from build123d import *

# Parameters (mm, degrees)
F0_W          = 203.2
F0_H          = 2032
F0_W_2        = 171.45
F0_H_2        = 320.1458333333
F1_DEPTH      = 22.225
F1_DEPTH_BACK = 22.225
F2_W          = 171.45
F2_H          = 320.1458333333
F3_DEPTH      = 21.59
F3_DEPTH_BACK = 21.59


with BuildPart() as f1:
    # F0 (on Front) → F1 (new body, two sides)
    with BuildSketch(Plane.XZ) as f1_sk:
        with Locations((101.6, 1016)):
            Rectangle(F0_W, F0_H)
        with Locations((101.6, 175.9479166667)):
            Rectangle(F0_W_2, F0_H_2, mode=Mode.SUBTRACT)
        with Locations((101.6, 511.96875)):
            Rectangle(F0_W_2, F0_H_2, mode=Mode.SUBTRACT)
        with Locations((101.6, 847.9895833333)):
            Rectangle(F0_W_2, F0_H_2, mode=Mode.SUBTRACT)
        with Locations((101.6, 1184.0104166667)):
            Rectangle(F0_W_2, F0_H_2, mode=Mode.SUBTRACT)
        with Locations((101.6, 1520.03125)):
            Rectangle(F0_W_2, F0_H_2, mode=Mode.SUBTRACT)
        with Locations((101.6, 1856.0520833333)):
            Rectangle(F0_W_2, F0_H_2, mode=Mode.SUBTRACT)
    extrude(amount=F1_DEPTH)
    extrude(f1_sk.sketch, amount=-F1_DEPTH_BACK)

    # F2 (on Front) → F3 (join, two sides)
    with BuildSketch(Plane.XZ) as f3_sk:
        with Locations((101.6, 1520.03125)):
            Rectangle(F2_W, F2_H)
        with BuildLine():
            Line((40.0148101771, 1504.2365351889), (122.7722068767, 1592.3491351889))
            ThreePointArc((122.7722068767, 1592.3491351889), (127.2601313551, 1592.4897903562), (127.4007865224, 1588.0018658778))
            Line((127.4007865224, 1588.0018658778), (44.6433898229, 1499.8892658778))
            ThreePointArc((44.6433898229, 1499.8892658778), (40.1554653445, 1499.7486107105), (40.0148101771, 1504.2365351889))
        make_face(mode=Mode.SUBTRACT)
        with BuildLine():
            ThreePointArc((158.5566101771, 1592.3491351889), (163.0445346555, 1592.4897903562), (163.1851898229, 1588.0018658778))
            Line((163.1851898229, 1588.0018658778), (44.6433898229, 1461.7892658778))
            ThreePointArc((44.6433898229, 1461.7892658778), (40.1554653445, 1461.6486107105), (40.0148101771, 1466.1365351889))
            Line((40.0148101771, 1466.1365351889), (158.5566101771, 1592.3491351889))
        make_face(mode=Mode.SUBTRACT)
        with BuildLine():
            Line((75.7992134776, 1466.1365351889), (158.5566101771, 1554.2491351889))
            ThreePointArc((158.5566101771, 1554.2491351889), (163.0445346555, 1554.3897903562), (163.1851898229, 1549.9018658778))
            Line((163.1851898229, 1549.9018658778), (80.4277931233, 1461.7892658778))
            ThreePointArc((80.4277931233, 1461.7892658778), (75.9398686449, 1461.6486107105), (75.7992134776, 1466.1365351889))
        make_face(mode=Mode.SUBTRACT)
        with Locations((101.6, 1184.0104166667)):
            Rectangle(F2_W, F2_H)
        with BuildLine():
            Line((40.0148101771, 1168.2156933889), (122.7722068767, 1256.3282933889))
            ThreePointArc((122.7722068767, 1256.3282933889), (127.2601313551, 1256.4689485562), (127.4007865224, 1251.9810240778))
            Line((127.4007865224, 1251.9810240778), (44.6433898229, 1163.8684240778))
            ThreePointArc((44.6433898229, 1163.8684240778), (40.1554653445, 1163.7277689105), (40.0148101771, 1168.2156933889))
        make_face(mode=Mode.SUBTRACT)
        with BuildLine():
            ThreePointArc((158.5566101771, 1256.3282933889), (163.0445346555, 1256.4689485562), (163.1851898229, 1251.9810240778))
            Line((163.1851898229, 1251.9810240778), (44.6433898229, 1125.7684240778))
            ThreePointArc((44.6433898229, 1125.7684240778), (40.1554653445, 1125.6277689105), (40.0148101771, 1130.1156933889))
            Line((40.0148101771, 1130.1156933889), (158.5566101771, 1256.3282933889))
        make_face(mode=Mode.SUBTRACT)
        with BuildLine():
            Line((75.7992134776, 1130.1156933889), (158.5566101771, 1218.2282933889))
            ThreePointArc((158.5566101771, 1218.2282933889), (163.0445346555, 1218.3689485562), (163.1851898229, 1213.8810240778))
            Line((163.1851898229, 1213.8810240778), (80.4277931233, 1125.7684240778))
            ThreePointArc((80.4277931233, 1125.7684240778), (75.9398686449, 1125.6277689105), (75.7992134776, 1130.1156933889))
        make_face(mode=Mode.SUBTRACT)
        with Locations((101.6, 847.9895833333)):
            Rectangle(F2_W, F2_H)
        with BuildLine():
            Line((40.0148101771, 832.1948515889), (122.7722068767, 920.3074515889))
            ThreePointArc((122.7722068767, 920.3074515889), (127.2601313551, 920.4481067562), (127.4007865224, 915.9601822778))
            Line((127.4007865224, 915.9601822778), (44.6433898229, 827.8475822778))
            ThreePointArc((44.6433898229, 827.8475822778), (40.1554653445, 827.7069271105), (40.0148101771, 832.1948515889))
        make_face(mode=Mode.SUBTRACT)
        with BuildLine():
            ThreePointArc((158.5566101771, 920.3074515889), (163.0445346555, 920.4481067562), (163.1851898229, 915.9601822778))
            Line((163.1851898229, 915.9601822778), (44.6433898229, 789.7475822778))
            ThreePointArc((44.6433898229, 789.7475822778), (40.1554653445, 789.6069271105), (40.0148101771, 794.0948515889))
            Line((40.0148101771, 794.0948515889), (158.5566101771, 920.3074515889))
        make_face(mode=Mode.SUBTRACT)
        with BuildLine():
            Line((75.7992134776, 794.0948515889), (158.5566101771, 882.2074515889))
            ThreePointArc((158.5566101771, 882.2074515889), (163.0445346555, 882.3481067562), (163.1851898229, 877.8601822778))
            Line((163.1851898229, 877.8601822778), (80.4277931233, 789.7475822778))
            ThreePointArc((80.4277931233, 789.7475822778), (75.9398686449, 789.6069271105), (75.7992134776, 794.0948515889))
        make_face(mode=Mode.SUBTRACT)
        with Locations((101.6, 511.96875)):
            Rectangle(F2_W, F2_H)
        with BuildLine():
            Line((40.0148101771, 496.1740097889), (122.7722068767, 584.2866097889))
            ThreePointArc((122.7722068767, 584.2866097889), (127.2601313551, 584.4272649562), (127.4007865224, 579.9393404778))
            Line((127.4007865224, 579.9393404778), (44.6433898229, 491.8267404778))
            ThreePointArc((44.6433898229, 491.8267404778), (40.1554653445, 491.6860853105), (40.0148101771, 496.1740097889))
        make_face(mode=Mode.SUBTRACT)
        with BuildLine():
            ThreePointArc((158.5566101771, 584.2866097889), (163.0445346555, 584.4272649562), (163.1851898229, 579.9393404778))
            Line((163.1851898229, 579.9393404778), (44.6433898229, 453.7267404778))
            ThreePointArc((44.6433898229, 453.7267404778), (40.1554653445, 453.5860853105), (40.0148101771, 458.0740097889))
            Line((40.0148101771, 458.0740097889), (158.5566101771, 584.2866097889))
        make_face(mode=Mode.SUBTRACT)
        with BuildLine():
            Line((75.7992134776, 458.0740097889), (158.5566101771, 546.1866097889))
            ThreePointArc((158.5566101771, 546.1866097889), (163.0445346555, 546.3272649562), (163.1851898229, 541.8393404778))
            Line((163.1851898229, 541.8393404778), (80.4277931233, 453.7267404778))
            ThreePointArc((80.4277931233, 453.7267404778), (75.9398686449, 453.5860853105), (75.7992134776, 458.0740097889))
        make_face(mode=Mode.SUBTRACT)
        Polygon((187.325, 336.0208333333), (15.875, 336.0208333333), (15.875, 15.875), (187.325, 15.875), (187.325, 246.0921333333), align=None)
        with BuildLine():
            Line((40.0148101771, 160.1531679889), (122.7722068767, 248.2657679889))
            ThreePointArc((122.7722068767, 248.2657679889), (127.2601313551, 248.4064231562), (127.4007865224, 243.9184986778))
            Line((127.4007865224, 243.9184986778), (44.6433898229, 155.8058986778))
            ThreePointArc((44.6433898229, 155.8058986778), (40.1554653445, 155.6652435105), (40.0148101771, 160.1531679889))
        make_face(mode=Mode.SUBTRACT)
        with BuildLine():
            ThreePointArc((158.5566101771, 248.2657679889), (162.0398214714, 249.0441237794), (164.0459, 246.0921333333))
            ThreePointArc((164.0459, 246.0921333333), (163.8228904461, 244.923211862), (163.1851898229, 243.9184986778))
            Line((163.1851898229, 243.9184986778), (44.6433898229, 117.7058986778))
            ThreePointArc((44.6433898229, 117.7058986778), (40.1554653445, 117.5652435105), (40.0148101771, 122.0531679889))
            Line((40.0148101771, 122.0531679889), (158.5566101771, 248.2657679889))
        make_face(mode=Mode.SUBTRACT)
        with BuildLine():
            Line((75.7992134776, 122.0531679889), (158.5566101771, 210.1657679889))
            ThreePointArc((158.5566101771, 210.1657679889), (163.0445346555, 210.3064231562), (163.1851898229, 205.8184986778))
            Line((163.1851898229, 205.8184986778), (80.4277931233, 117.7058986778))
            ThreePointArc((80.4277931233, 117.7058986778), (75.9398686449, 117.5652435105), (75.7992134776, 122.0531679889))
        make_face(mode=Mode.SUBTRACT)
        with Locations((101.6, 1856.0520833333)):
            Rectangle(F2_W, F2_H)
        with BuildLine():
            Line((40.0148101771, 1840.2573769889), (122.7722068767, 1928.3699769889))
            ThreePointArc((122.7722068767, 1928.3699769889), (127.2601313551, 1928.5106321562), (127.4007865224, 1924.0227076778))
            Line((127.4007865224, 1924.0227076778), (44.6433898229, 1835.9101076778))
            ThreePointArc((44.6433898229, 1835.9101076778), (40.1554653445, 1835.7694525105), (40.0148101771, 1840.2573769889))
        make_face(mode=Mode.SUBTRACT)
        with BuildLine():
            ThreePointArc((158.5566101771, 1928.3699769889), (163.0445346555, 1928.5106321562), (163.1851898229, 1924.0227076778))
            Line((163.1851898229, 1924.0227076778), (44.6433898229, 1797.8101076778))
            ThreePointArc((44.6433898229, 1797.8101076778), (40.1554653445, 1797.6694525105), (40.0148101771, 1802.1573769889))
            Line((40.0148101771, 1802.1573769889), (158.5566101771, 1928.3699769889))
        make_face(mode=Mode.SUBTRACT)
        with BuildLine():
            Line((75.7992134776, 1802.1573769889), (158.5566101771, 1890.2699769889))
            ThreePointArc((158.5566101771, 1890.2699769889), (163.0445346555, 1890.4106321562), (163.1851898229, 1885.9227076778))
            Line((163.1851898229, 1885.9227076778), (80.4277931233, 1797.8101076778))
            ThreePointArc((80.4277931233, 1797.8101076778), (75.9398686449, 1797.6694525105), (75.7992134776, 1802.1573769889))
        make_face(mode=Mode.SUBTRACT)
    extrude(amount=F3_DEPTH)
    extrude(f3_sk.sketch, amount=-F3_DEPTH_BACK)


solid = f1.part
The listing builds one solid part. Answer for the finished solid, in the listing's coordinates (mm). A direction names the side the tool comes from. Give positions to 0.01 mm unless a question says otherwise; leave off trailing zeros. Write each loop counter-clockwise with the first axis right and the second up, starting at its lowest first coordinate (ties: lowest second). Pieces come first, ordered by that corner, then holes.
Item 1: Which of the six approach directions +Z, -Z, +X, -X, +Y, -Y give full straight-line access (tool end or side, diameter ignored) to faces 1 (the flat face through (86.6, -0.3, 1544.56)), 2 (the flat face through (203.2, 0, 1002))?
Item 2: Flat-ended cylindrical pins translate along their axes: P1, Ø0.5, axis at x = 118, y = 22, coming from the -Z side; P2, Ø3, axis at x = 183, z = 1662.5, coming from the +Y side; P3, Ø4, axis at x = 121, z = 1240, coming from the -Y side. Find the tip coordinate at first contact, or state that the pin passes through.
Item 3: Section B-B, the plane y = 6 is taken. Count the separate pieces of the cut face and the enclosed holes in it, plus the area to 3 significant figures.
Item 4: Section A-A, the plane z = 1067 is taken. Write down the section's boundary in (x, y) (3 decimals).
Item 5: Find the intervals of material crossed by line 1 along X through (y, z) = (2.5, 791); line 2 along X through (y, z) = (-6, 144.5); line 3 along X through (y, z) = (-0.5, 493.5), in increasing order.
Completed:
1. face 1: +Y, -Y
1. face 2: +Z, -Z, +X, +Y, -Y
2. P1: stops at z = 0
2. P2: stops at y = 21.59
2. P3: stops at y = -21.59
3. separate pieces: 1
3. enclosed holes: 18
3. area: 397,000 mm2
4. outline: (0, -22.225) - (15.875, -22.225) - (15.875, -21.59) - (187.325, -21.59) - (187.325, -22.225) - (203.2, -22.225) - (203.2, 22.225) - (187.325, 22.225) - (187.325, 21.59) - (15.875, 21.59) - (15.875, 22.225) - (0, 22.225) - close
5. line 1: x = 0 to 39.29, 45.82 to 75.08, 81.6 to 203.2
5. line 2: x = 0 to 61.1, 69.81 to 96.88, 105.59 to 203.2
5. line 3: x = 0 to 39.19, 46.21 to 73.29, 82 to 109.07, 117.78 to 203.2
